Autodesk Inventor part; units mm, degrees
ref_plane "YZ Plane" through (0, 0, 0) normal (1, 0, 0) x (0, 1, 0)
ref_plane "XY Plane" through (0, 0, 0) normal (0, 0, 1) x (1, 0, 0)
ref_plane "Arbeitsebene1" through (0, 0, 10) normal (0, 0, 1) x (1, 0, 0)
sketch "Skizze1" plane through (0, 0, 10) normal (0, 0, 1) x (1, 0, 0)
  circle A0 centre (19.3, 0) radius 19.3
  circle A1 centre (5.0106, 8.25) radius 1.4
  circle A2 centre (33.5894, 8.25) radius 1.4
  circle A3 centre (19.3, -16.5) radius 1.5
  circle A4 centre (19.3, 0) radius 2.15
  point P0 (0, 0)
  dimension "d0" = 4.3
extrude "Extrusion1" add sketch "Skizze1" along normal blind 1.5
sketch "Skizze2" plane through (19.3, 0, 10) normal (0, 0, -1) x (-1, 0, 0)
  circle A0 centre (0, 0) radius 2.15
  circle A1 centre (0, 0) radius 5.3
  circle A2 centre (0, 0) radius 19.3
  circle A3 centre (0, 0) radius 2.15
  circle A4 centre (0, -16.5) radius 1.5
  circle A5 centre (-14.2894, 8.25) radius 1.4
  circle A6 centre (14.2894, 8.25) radius 1.4
  circle A7 centre (0, 0) radius 5.8
  circle A8 centre (0, 0) radius 8
  circle A9 centre (0, 0) radius 2.65
  point P0 (19.3, 0)
  dimension "d6" = 10.6
  dimension "d7" = 0.5
  dimension "d8" = 16
  dimension "d13" = 0.5
extrude "Extrusion2" add sketch "Skizze2" along normal blind 3 contours A2 | A7 | A8 | A9
sketch "Skizze3" plane through (0, 0, 0) normal (0, 1, 0) x (-1, 0, 0)
  point P0 (0, 0)
ref_plane "Arbeitsebene2" through (0, 5, 0) normal (0, 1, 0) x (-1, 0, 0)
properties part number "50_ETL_Top_Seal_v1"
Verification items for the finished model (mm, model axes). A direction names the side the tool comes from. Coordinates: 2 decimals unless noted, no trailing zeros. Order: outer loops, then holes, each group sorted by start corner. A loop starts at its lowest first (then second) coordinate and runs counter-clockwise, first axis right, second up.
1. Release check for a two-part mould opening along X. For faces 1 (the face through (23, 0, 11.5)), 2 (the face through (21.947, -0.117, 8.521)) record: +X half, -X half, draft (parallel to the pull), parting line (faces both ways), or undercut.
Results found:
face 1: draft
face 2: undercut
2. Sectioned sample at A-A, the plane z = 8.1. Record the cut outline in (x, y), and give its area (3 significant figures).
Results found:
outline: circle Ø38.6 at (19.3, 0); circle Ø5.3 at (19.3, 0); hole circle Ø2.8 at (5.01, 8.25); hole circle Ø10.6 at (19.3, 0); hole circle Ø4.3 at (19.3, 0); hole circle Ø3 at (19.3, -16.5); hole circle Ø2.8 at (33.59, 8.25)
area: 1,070 mm2
3. Scan lines: line 1 (Y direction, x = 19.3, z = 9.3); line 2 (Y direction, x = 19.3, z = 10.9); line 3 (Y direction, x = 21, z = 7.2). Record each from-to range of solid material in increasing order.
Results found:
line 1: y = -19.3 to -18, -15 to -5.3, -2.65 to -2.15, 2.15 to 2.65, 5.3 to 19.3
line 2: y = -19.3 to -18, -15 to -2.15, 2.15 to 19.3
line 3: y = -19.22 to -5.02, -2.03 to -1.32, 1.32 to 2.03, 5.02 to 19.22
4. Set-up check for faces 3 (the face through (22, -2, 10)), 4 (the face through (15, -4, 7)): record each of +Z, -Z, +X, -X, +Y, -Y from which the full face is reachable in a straight line by a thin tool's end or side.
Results found:
face 3: -Z
face 4: -Z, +X, -X, +Y, -Y
5. Sectioned sample at D-D, the plane y = 8.25. Record the cut outline in (x, z).
Results found:
outline: (1.85, 7) - (3.61, 7) - (3.61, 11.5) - (1.85, 11.5) - close; (6.41, 7) - (32.19, 7) - (32.19, 11.5) - (6.41, 11.5) - close; (34.99, 7) - (36.75, 7) - (36.75, 11.5) - (34.99, 11.5) - close
6. Sectioned sample at C-C, the plane x = 19.3. Record the cut outline in (y, z).
Results found:
outline: (-19.3, 7) - (-18, 7) - (-18, 11.5) - (-19.3, 11.5) - close; (-15, 7) - (-5.3, 7) - (-5.3, 10) - (-2.65, 10) - (-2.65, 7) - (-2.15, 7) - (-2.15, 11.5) - (-15, 11.5) - close; (2.15, 7) - (2.65, 7) - (2.65, 10) - (5.3, 10) - (5.3, 7) - (19.3, 7) - (19.3, 11.5) - (2.15, 11.5) - close
7. Sectioned sample at B-B, the plane y = 0. Record the cut outline in (x, z), and give its area (3 significant figures).
Results found:
outline: (0, 7) - (14, 7) - (14, 10) - (16.65, 10) - (16.65, 7) - (17.15, 7) - (17.15, 11.5) - (0, 11.5) - close; (21.45, 7) - (21.95, 7) - (21.95, 10) - (24.6, 10) - (24.6, 7) - (38.6, 7) - (38.6, 11.5) - (21.45, 11.5) - close
area: 138 mm2
